Solid Edge part; units mm, degrees
sketch "Sketch1" plane through (0, 0, 0) normal (0, -1, 0) x (1, 0, 0)
  line L0 (0, 12) -> (45, 12)
  line L1 (45, 12) -> (45, 0)
  line L2 (35, 0) -> (45, 0)
  line L3 (35, 3) -> (35, 0)
  line L4 (10, 3) -> (35, 3)
  line L5 (10, 0) -> (10, 3)
  line L6 (0, 0) -> (10, 0)
  line L7 (0, 0) -> (0, 12)
  line L8 (166, 12) -> (121, 12)
  line L9 (121, 12) -> (121, 0)
  line L10 (121, 0) -> (131, 0)
  line L11 (131, 0) -> (131, 3)
  line L12 (131, 3) -> (156, 3)
  line L13 (156, 3) -> (156, 0)
  line L14 (156, 0) -> (166, 0)
  line L15 (166, 0) -> (166, 12)
extrude "Protrusion1" add sketch "Sketch1" against normal blind 76
sketch "Sketch2" plane through (143.5, 38, 12) normal (0, 0, 1) x (1, 0, 0)
  line L0 (-12.5, -28) -> (-12.5, 28)
  line L1 (-12.5, 28) -> (-22.5, 28)
  line L2 (-22.5, 28) -> (-22.5, -28)
  line L3 (-22.5, -28) -> (-12.5, -28)
  line L4 (-108.5, -28) -> (-108.5, 28)
  line L5 (-108.5, 28) -> (-98.5, 28)
  line L6 (-98.5, 28) -> (-98.5, -28)
  line L7 (-98.5, -28) -> (-108.5, -28)
extrude "ExtrudedProtrusion_2" add sketch "Sketch2" along normal blind 76
sketch "Sketch3" plane through (131, 38, 50) normal (1, 0, 0) x (0, 1, 0)
  line L0 (28, 38) -> (-28, 38)
  line L1 (-28, 38) -> (-28, 28)
  line L2 (-28, 28) -> (28, 28)
  line L3 (28, 28) -> (28, 38)
extrude "ExtrudedProtrusion_3" add sketch "Sketch3" against normal blind 96
sketch "Sketch4" plane through (83, 38, 88) normal (0, 0, 1) x (0, 1, 0)
  circle A0 centre (0, 0) radius 12.5
  circle A1 centre (0, 0) radius 25
extrude "ExtrudedProtrusion_4" add sketch "Sketch4" along normal blind 25
fillet "Round_1" radius 10 6 edges at (131, 38, 88) (126, 66, 12) (40, 66, 12) (35, 38, 88) (40, 10, 12) (126, 10, 12)
The model under review builds one solid part; all positions refer to its coordinate system, in mm. A direction names the side the tool comes from. Give positions to 0.01 mm unless a question says otherwise; leave off trailing zeros. Loops run counter-clockwise (first coordinate to the right, second up) from the corner with the lowest first, then second, coordinate; pieces in that order, holes last. Notation, with made-up numbers: (34.25, 52) -> (54.25, 52) arc R27 ccw to (54.25, 79) -> close; hole circle Ø5 at (22, 21). An arc over 180 degrees is marked (long way). Put each result on its own line as item: value. Start each with the question number.
1. Clearance check with flat-ended pins moving along their axes: P1, Ø7.5, axis at x = 145.5, y = 41, coming from the -Z side; P2, Ø17, axis at x = 71.5, y = 40.5, coming from the -Z side; P3, Ø2, axis at y = 52.5, z = 20, coming from the -X side. State where each tip first meets the part, or that it passes through.
2. Wall thickness on probe 1 along Y at (x, z) = (83, 104); probe 2 along X at (y, z) = (38, 98); probe 3 along X at (y, z) = (28.5, 49): over which ranges is each line inside the solid? List them lowest first.
3. We need section D-D on y = 5.5. State the section outline as (x, z) points, then the cut area to 3 significant figures.
4. For faces 5 (the face through (73.42, 61.09, 100.32)), 6 (the face through (45, 37, 40)), 7 (the face through (35, 37, 45)), list the 3-axis set-ups (+Z, -Z, +X, -X, +Y, -Y) from which the entire face can be reached by the end or side of a thin tool; tool diameter is ignored.
5. We need section C-C on x = 83. State the section outline as (y, z) points, then the cut area to 4 significant figures.
6. We need section A-A on z = 58. State the section outline as (x, y) points, then the cut area to 3 significant figures.
7. Mouldability with a two-part tool opening along Y and no side actions: class faces 1 (the face through (127.99, 38.39, 85.15)), 2 (the face through (23, 76, 6)), 3 (the face through (83, 38, 88)), 4 (the face through (95.394, 36.373, 100.325)) as released by +Y, released by -Y, zero draft, split by the parting line, or undercut.
Determined:
1. P1: z = 3
1. P2: z = 78
1. P3: x = 35
2. probe 1: 13 to 25.5, 50.5 to 63
2. probe 2: 58 to 70.5, 95.5 to 108
2. probe 3: 35 to 45, 121 to 131
3. outline: (0, 0) -> (10, 0) -> (10, 3) -> (35, 3) -> (35, 0) -> (45, 0) -> (45, 13.65) -> (35, 13.65) -> (35, 12) -> (0, 12) -> close; (121, 0) -> (131, 0) -> (131, 3) -> (156, 3) -> (156, 0) -> (166, 0) -> (166, 12) -> (131, 12) -> (131, 13.65) -> (121, 13.65) -> close
3. area: 963 mm^2
4. face 5: +Z
4. face 6: -Z, +Y, -Y
4. face 7: +Z, -X, +Y, -Y
5. outline: (10, 78) -> (66, 78) -> (66, 88) -> (63, 88) -> (63, 113) -> (50.5, 113) -> (50.5, 88) -> (25.5, 88) -> (25.5, 113) -> (13, 113) -> (13, 88) -> (10, 88) -> close
5. area: 1,185 mm^2
6. outline: (35, 10) -> (45, 10) -> (45, 66) -> (35, 66) -> close; (121, 10) -> (131, 10) -> (131, 66) -> (121, 66) -> close
6. area: 1,120 mm^2
7. face 1: zero draft
7. face 2: released by +Y
7. face 3: undercut
7. face 4: undercut
